from build123d import *

# Parameters (mm, degrees)
EXTRUDE_1_DEPTH           = 2.75
SKETCH_2_W                = 2.6
SKETCH_2_H                = 1.5
HOLE_WIZARD_3_0_3_1_D     = 3
HOLE_WIZARD_3_0_3_1_DEPTH = 4.25
FILLET_1_R                = 1


with BuildPart() as part:
    # 草图1 → 凸台-拉伸1 (new body)
    with BuildSketch(Plane.XY.offset(2.75)):
        Polygon((1.58771324, -2.75), (3.175426481, 0), (1.58771324, 2.75), (-1.58771324, 2.75), (-3.175426481, 0), (-1.58771324, -2.75), align=None)
    extrude(amount=-EXTRUDE_1_DEPTH)

    # 草图2 → 旋转1 (revolve)
    with BuildSketch(Plane(origin=(0, 0, 0), x_dir=(1, 0, 0), z_dir=(0, 1, 0))):
        with Locations((1.3, -3.5)):
            Rectangle(SKETCH_2_W, SKETCH_2_H)
    revolve(axis=Axis((0, 0, 2.75), (0, 0, 1)))

    # Ø3.0 (3) 直径孔1
    with Locations(Plane(origin=(0, 0, 0), x_dir=(-1, 0, 0), z_dir=(0, 0, -1))):
        with Locations((0, 0)):
            Hole(HOLE_WIZARD_3_0_3_1_D / 2, depth=HOLE_WIZARD_3_0_3_1_DEPTH)

    # 圆角1
    fillet_1_edges = [part.edges().sort_by_distance(p)[0] for p in [
        (-2.6, 0, 4.25),
    ]]
    fillet(fillet_1_edges, radius=FILLET_1_R)


solid = part.part
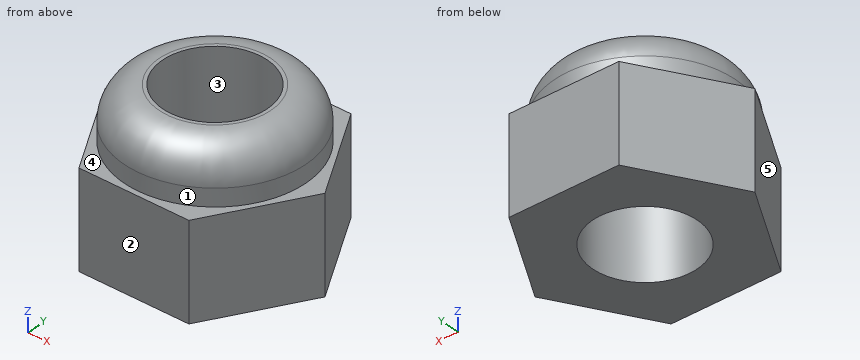
Geometry check sheet. Reference: the model listing, model coordinates, mm. Face numbers are marked on the shaded views. A direction names the side the tool comes from. Give positions to 0.01 mm unless a question says otherwise; leave off trailing zeros. Loops run counter-clockwise (first coordinate to the right, second up) from the corner with the lowest first, then second, coordinate; pieces in that order, holes last. Notation, with made-up numbers: (58.5, 57) -> (98.5, 57) arc R34 cw to (98.5, 95) -> close; hole circle Ø2 at (24, 49). An arc over 180 degrees is marked (long way). Answer in a Markdown table with one row per item. Add a question column.
1) Set-up check for the marked faces 4 and 5: record each of +Z, -Z, +X, -X, +Y, -Y from which the full face is reachable in a straight line by a thin tool's end or side.
2) Gauge pin test, flat end, axial feed: P1, Ø2, axis at y = -2, z = 2, coming from the +X side. Record the tip position at first contact, or that the pin passes through.
3) Draft check along Y on the marked faces 1, 2 and 3. Enter one of: pulls with the +Y half, pulls with the -Y half, needs draft (parallel to the pull), parting line crosses it, or undercut.
4) Material ranges on probe 1 along Y at (x, z) = (0, 2.2); probe 2 along X at (y, z) = (-0.95, 4); probe 3 along X at (y, z) = (0.9, 0.5), recorded low to high. Write a range as from..to.
5) Cross-section at C-C on x = 2.75. Record the boundary of the cut face in (y, z).
6) Cross-section at B-B on z = 3.85. Record the boundary of the cut face in (x, y), and give its area (3 significant figures).
7) Cross-section at A-A on x = 0. Record the boundary of the cut face in (y, z).
Outcome:
| question | item | result |
|---|---|---|
| 1 | face 4 | +Z |
| 1 | face 5 | +Z, -Z, -X, -Y |
| 2 | P1 | stops at x = 2.6 |
| 3 | face 1 | parting line crosses it |
| 3 | face 2 | pulls with the -Y half |
| 3 | face 3 | undercut |
| 4 | probe 1 | y = -2.75..-1.5, 1.5..2.75 |
| 4 | probe 2 | x = -2.05..-1.16, 1.16..2.05 |
| 4 | probe 3 | x = -2.66..-1.2, 1.2..2.66 |
| 5 | outline | (-0.74, 0) -> (0.74, 0) -> (0.74, 2.75) -> (-0.74, 2.75) -> close |
| 6 | outline | circle Ø4.8 at (0, 0); hole circle Ø3 at (0, 0) |
| 6 | area | 11.0 mm^2 |
| 7 | outline | (-2.75, 0) -> (-1.5, 0) -> (-1.5, 4.25) -> (-1.6, 4.25) arc R1 ccw to (-2.6, 3.25) -> (-2.6, 2.75) -> (-2.75, 2.75) -> close; (1.5, 0) -> (2.75, 0) -> (2.75, 2.75) -> (2.6, 2.75) -> (2.6, 3.25) arc R1 ccw to (1.6, 4.25) -> (1.5, 4.25) -> close |
